For this review, take the finished solid that the model builds, in its own axes (mm). A direction names the side the tool comes from. Give positions to 0.01 mm unless a question says otherwise; leave off trailing zeros. Write each loop counter-clockwise with the first axis right and the second up, starting at its lowest first coordinate (ties: lowest second). Pieces come first, ordered by that corner, then holes. Notation, with made-up numbers: (29, -9.75) -> (56, -9.75) arc R21 cw to (56, 24.25) -> close; hole circle Ø7 at (-33.75, 5.25). An arc over 180 degrees is marked (long way). Answer as CSV lines item,"result".
Autodesk Fusion 360 part; units mm, degrees
sketch "Sketch1" plane through (0, 0, 0) normal (0, 1, 0) x (1, 0, 0)
  line L0 (3.75, -19.5) -> (-3.75, -19.5)
  line L1 (-3.75, -19.5) -> (-3.75, 19.5)
  line L2 (-3.75, 19.5) -> (3.75, 19.5)
  line L3 (3.75, 19.5) -> (3.75, -19.5)
  line L4 (3.75, -19.5) -> (-3.75, 19.5) construction
  line L5 (-3.75, -19.5) -> (3.75, 19.5) construction
  circle A0 centre (66.05, 0) radius 15
  line L6 (3.75, -19.5) -> (67.1215, -14.9617)
  line L7 (3.75, 19.5) -> (67.1215, 14.9617)
  dimension "d1" = 7.5
  dimension "d2" = 39
  dimension "d4" = 30
extrude "Extrude1" add sketch "Sketch1" along normal blind 7
sketch "Sketch2" plane through (0, 7, 0) normal (0, 1, 0) x (-1, 0, 0)
  line L0 (-3.75, 19.5) -> (-67.1215, 14.9617)
  arc A0 (-67.1215, 14.9617) -> (-67.1215, -14.9617) centre (-66.05, 0) ccw
  line L1 (-67.1215, -14.9617) -> (-3.75, -19.5)
  line L2 (-3.75, -19.5) -> (3.75, -19.5)
  line L3 (3.75, -19.5) -> (3.75, 19.5)
  line L4 (3.75, 19.5) -> (-3.75, 19.5)
  line L5 (3.75, -19.5) -> (-3.75, -19.5)
  line L6 (-3.75, -19.5) -> (-3.75, 19.5)
  line L7 (-3.75, 19.5) -> (3.75, 19.5)
  line L8 (3.75, 19.5) -> (3.75, -19.5)
extrude "Extrude2" add sketch "Sketch2" against normal blind 23.35 contours L2 L3 L4 L5 L6 L7 L8
sketch "Sketch3" plane through (0, 0, -19.5) normal (0, 0, -1) x (-1, 0, 0)
  line L0 (3.75, -16.35) -> (3.75, 7)
  line L1 (3.75, 7) -> (-3.75, 7)
  line L2 (-3.75, 7) -> (-3.75, 0)
  line L3 (-3.75, 0) -> (-3.75, -16.35)
  line L4 (-3.75, -16.35) -> (3.75, -16.35)
  line L5 (3.75, -16.35) -> (3.75, -19.22)
  line L6 (3.75, -19.22) -> (-3.75, -16.35)
  dimension "d9" = 2.87
extrude "Extrude3" add sketch "Sketch3" against normal blind 39 contours L4 L5 L6
sketch "Sketch4" plane through (0, 0, 0) normal (0, -1, 0) x (1, 0, 0)
  line L0 (3.75, 19.5) -> (3.75, -19.5)
  line L1 (3.75, -19.5) -> (67.1215, -14.9617)
  arc A0 (67.1215, -14.9617) -> (67.1215, 14.9617) centre (66.05, 0) ccw
  line L2 (67.1215, 14.9617) -> (3.75, 19.5)
  line L3 (3.75, -19.5) -> (17.7142, -18.5)
  line L4 (17.7142, -18.5) -> (23.6989, -18.0714)
  line L5 (3.75, 19.5) -> (17.7142, 18.5)
  line L6 (17.7142, 18.5) -> (23.6989, 18.0714)
  line L7 (23.6989, 18.0714) -> (23.6989, -18.0714)
  line L8 (17.7142, 18.5) -> (17.7142, -18.5)
  dimension "d12" = 14
  dimension "d13" = 6
  dimension "d14" = 14
  dimension "d15" = 6
extrude "Extrude4" add sketch "Sketch4" along normal blind 53.35 contours L1 L2 L4 L6 L7 L8
sketch "Sketch5" plane through (23.6989, 0, 0) normal (1, 0, 0) x (0, 0, -1)
  line L0 (18.0714, 0) -> (-18.0714, 0)
  line L1 (-18.0714, 0) -> (-18.0714, -53.35)
  line L2 (-18.0714, -53.35) -> (18.0714, -53.35)
  line L3 (18.0714, -53.35) -> (18.0714, 0)
  line L4 (-11.0714, -48.35) -> (8.6618, -48.35)
  line L5 (11.0714, -5) -> (-8.6618, -5)
  line L6 (13.0714, -7) -> (13.0714, -17.5)
  line L7 (11.64, -16.8156) -> (-9.0931, -6.9022)
  line L8 (-13.0714, -46.35) -> (-13.0714, -35.85)
  line L9 (9.0931, -46.4478) -> (-11.64, -36.5344)
  line L10 (10.9243, -39.8234) -> (-10.2282, -29.7094)
  line L11 (-10.9243, -13.5266) -> (10.2282, -23.6406)
  line L12 (13.0714, -38.4701) -> (13.0714, -28.1514)
  line L13 (13.0714, -15.9134) -> (13.0714, -5)
  line L14 (-13.0714, -14.8799) -> (-13.0714, -25.1986)
  line L15 (-13.0714, -37.4366) -> (-13.0714, -48.35)
  arc A0 (8.6618, -48.35) -> (9.0931, -46.4478) centre (8.6618, -47.35) ccw
  arc A1 (-11.64, -36.5344) -> (-13.0714, -37.4366) centre (-12.0714, -37.4366) ccw
  arc A2 (11.64, -16.8156) -> (13.0714, -15.9134) centre (12.0714, -15.9134) ccw
  arc A3 (-8.6618, -5) -> (-9.0931, -6.9022) centre (-8.6618, -6) ccw
  arc A4 (13.0714, -7) -> (11.0714, -5) centre (11.0714, -7) ccw
  arc A5 (-13.0714, -46.35) -> (-11.0714, -48.35) centre (-11.0714, -46.35) ccw
  arc A6 (10.9243, -39.8234) -> (13.0714, -38.4701) centre (11.5714, -38.4701) ccw
  arc A7 (-10.9243, -13.5266) -> (-13.0714, -14.8799) centre (-11.5714, -14.8799) ccw
  arc A8 (13.0714, -28.1514) -> (10.2282, -23.6406) centre (8.0714, -28.1514) ccw
  arc A9 (-13.0714, -25.1986) -> (-10.2282, -29.7094) centre (-8.0714, -25.1986) ccw
  point P0 (-13.0714, -5)
  point P1 (13.0714, -48.35)
  point P2 (13.0714, -25)
  point P3 (-13.0714, -28.35)
  point P4 (13.0714, -40.85)
  point P5 (-13.0714, -12.5)
  dimension "d19" = 12.5
  dimension "d20" = 7.5
  dimension "d21" = 12.5
  dimension "d22" = 7.5
  dimension "d23" = 7.5
  dimension "d24" = 7.5
  dimension "d25" = 1
  dimension "d26" = 2
  dimension "d27" = 1.5
  dimension "d28" = 5
extrude "Extrude5" cut sketch "Sketch5" against normal blind 9 contours L4 L8 L9 L15 A0 A1 A5 | L5 L6 L7 L13 A2 A3 A4 | L10 L11 L12 L14 A6 A7 A8 A9
sketch "Sketch6" plane through (0, 0, 0) normal (0, -1, 0) x (1, 0, 0)
  line L0 (23.6989, 18.0714) -> (23.6989, -18.0714)
  line L1 (23.6989, -18.0714) -> (67.1215, -14.9617)
  arc A0 (67.1215, -14.9617) -> (67.1215, 14.9617) centre (66.05, 0) ccw
  line L2 (67.1215, 14.9617) -> (23.6989, 18.0714)
  circle A1 centre (66.05, 0) radius 10.35
  dimension "d31" = 20.7
extrude "Extrude6" cut sketch "Sketch6" against normal blind 1.6 contours A1
sketch "Sketch7" plane through (0, 1.6, 0) normal (0, -1, 0) x (1, 0, 0)
  circle A0 centre (66.05, 0) radius 10.35
  circle A1 centre (66.05, 0) radius 1.6
  line L0 (66.05, 0) -> (59.05, 0)
  line L1 (66.05, 0) -> (73.05, 0)
  line L2 (66.05, 0) -> (66.05, -7)
  line L3 (66.05, 0) -> (66.05, 7)
  circle A2 centre (59.05, 0) radius 0.75
  circle A3 centre (66.05, 7) radius 0.75
  circle A4 centre (73.05, 0) radius 0.75
  circle A5 centre (66.05, -7) radius 0.75
  dimension "d34" = 3.2
  dimension "d35" = 7
  dimension "d36" = 7
  dimension "d37" = 7
  dimension "d38" = 7
  dimension "d39" = 1.5
  dimension "d40" = 1.5
  dimension "d41" = 1.5
  dimension "d42" = 1.5
extrude "Extrude7" cut sketch "Sketch7" against normal blind 13 contours A1 L1 L3 | A5 | A2 | A3 | A1 L1 L2 | A4 | A1 L0 L3 | A1 L0 L2
sketch "Sketch8" plane through (3.75, 0, 0) normal (1, 0, 0) x (0, 0, -1)
  line L0 (19.5, 0) -> (-19.5, 0)
  line L1 (-19.5, 0) -> (-19.5, -16.35)
  line L2 (-19.5, -16.35) -> (19.5, -16.35)
  line L3 (19.5, -16.35) -> (19.5, 0)
  line L4 (19.5, -16.35) -> (10, -16.35)
  line L5 (10, -16.35) -> (10, -11.35)
  circle A0 centre (10, -11.35) radius 1.6
  line L6 (10, -11.35) -> (-10, -11.35)
  circle A1 centre (-10, -11.35) radius 1.6
  dimension "d45" = 9.5
  dimension "d46" = 5
  dimension "d47" = 3.2
  dimension "d48" = 20
  dimension "d49" = 3.2
extrude "Extrude8" cut sketch "Sketch8" against normal blind 19 contours A1 | L5 A0 L6 | L5 A0 L6
sketch "Sketch9" plane through (0, -53.35, 0) normal (0, -1, 0) x (1, 0, 0)
  line L0 (23.6989, 18.0714) -> (17.7142, 18.5)
  line L1 (17.7142, 18.5) -> (17.7142, -18.5)
  line L2 (17.7142, -18.5) -> (23.6989, -18.0714)
  line L3 (23.6989, -18.0714) -> (23.6989, 18.0714)
  circle A0 centre (20.7416, 0) radius 1.6
  circle A1 centre (20.7416, 10) radius 1.6
  circle A2 centre (20.7416, -10) radius 1.6
  dimension "d52" = 3.2
  dimension "d53" = 10
  dimension "d54" = 10
  dimension "d55" = 3.2
  dimension "d56" = 3.2
extrude "Extrude9" cut sketch "Sketch9" against normal blind 4 contours A0 | A1 | A2
Q1. Clearance check with flat-ended pins moving along their axes: pin 1 (4 mm diameter, centred on x = 66.05, z = 0, fed in from -Y); pin 2 (1.5 mm diameter, centred on y = -17.5, z = 14, fed in from +X); pin 3 (6.5 mm diameter, centred on x = 22, y = -34.5, fed in from +Z). State where each tip first meets the part, or that it passes through.
Answer block:
pin 1,"stops at y = 1.6"
pin 2,"stops at x = 23.7"
pin 3,"stops at z = 18.43"
Q2. Add section B-B (y = -21). Write out the cut boundary in (x, z).
Answer block:
outline,"(17.71, -18.5) -> (23.7, -18.07) -> (23.7, -4.71) -> (17.71, -4.71) -> close; (17.71, 13.07) -> (23.7, 13.07) -> (23.7, 18.07) -> (17.71, 18.5) -> close"
Q3. Add section D-D (x = 30). Write out the cut boundary in (y, z).
Answer block:
outline,"(0, -17.62) -> (7, -17.62) -> (7, 17.62) -> (0, 17.62) -> close"
Q4. For faces 1 (the flat face through (17.714, -20, -4)), 2 (the cylindrical face through (55.71, 0.79, 0.46)), 3 (the flat face through (21, -33, -13.071)), list the 3-axis set-ups (+Z, -Z, +X, -X, +Y, -Y) from which the entire face can be reached by the end or side of a thin tool; tool diameter is ignored.
Answer block:
face 1,"+Z, -Z, -Y"
face 2,"-Y"
face 3,"+X, -X"
Q5. Draft analysis for pull direction X (two halves, no side actions). For faces 4 (the cylindrical face through (20.748, -5.761, 9.633)), 5 (the cylindrical face through (21.48, -51.38, -11.42)), 6 (the flat face through (23.699, -20, -4)), 7 (the flat face through (66, 1.6, -2)), state which applies: released by +X, released by -X, zero draft, split by the parting line, or undercut.
Answer block:
face 4,"zero draft"
face 5,"undercut"
face 6,"released by +X"
face 7,"undercut"
Q6. Add section A-A (y = -11.35). Write out the cut boundary in (x, z).
Answer block:
outline,"(-3.75, -19.5) -> (3.75, -19.5) -> (3.75, -11.6) -> (-3.75, -11.6) -> close; (-3.75, -8.4) -> (3.75, -8.4) -> (3.75, 8.4) -> (-3.75, 8.4) -> close; (-3.75, 11.6) -> (3.75, 11.6) -> (3.75, 19.5) -> (-3.75, 19.5) -> close; (17.71, -18.5) -> (23.7, -18.07) -> (23.7, -13.07) -> (17.71, -13.07) -> close; (17.71, -0.21) -> (23.7, -0.21) -> (23.7, 18.07) -> (17.71, 18.5) -> close"
Q7. Add section C-C (x = 75). Write out the cut boundary in (y, z), plus the area to 3 significant figures.
Answer block:
outline,"(0, -12.04) -> (7, -12.04) -> (7, 12.04) -> (0, 12.04) -> (0, 5.2) -> (1.6, 5.2) -> (1.6, -5.2) -> (0, -5.2) -> close"
area,"152 mm2"
Q8. To check wall thickness, follow probe 1 along X at (y, z) = (1.5, -0.5); probe 2 along X at (y, z) = (-14.5, -14); probe 3 along Y at (x, z) = (53, 4.5). State the ranges of each line that lie inside material, in increasing order. Write a range as [from, to].
Answer block:
probe 1,"x = [-3.75, 55.71], [76.39, 81.04]"
probe 2,"x = [-3.75, 3.75], [17.71, 23.7]"
probe 3,"y = [0, 7]"
